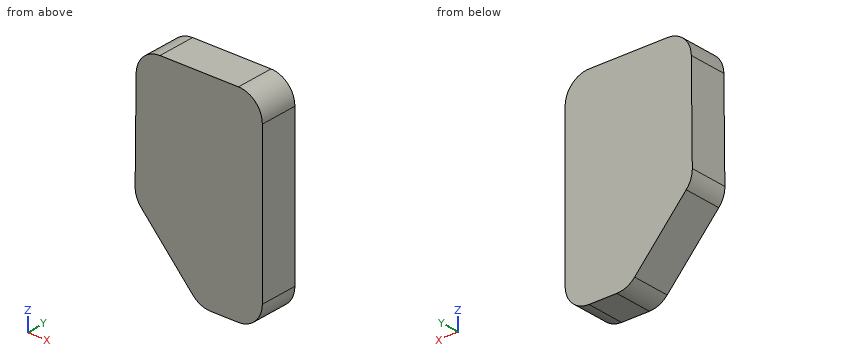
```python
from build123d import *

# Parameters (mm, degrees)
ESQUISSE1_W             = 80
ESQUISSE1_H             = 16
BOSS_EXTRU_1_DEPTH      = 85
ENL_V_MAT_EXTRU_1_DEPTH = 118.817655723
CONG_1_R                = 10
ENL_V_MAT_EXTRU_2_DEPTH = 118.817655723
CONG_2_R                = 10


with BuildPart() as part:
    # Esquisse1 → Boss.-Extru.1 (new body)
    with BuildSketch(Plane.XY):
        with Locations((40, 8)):
            Rectangle(ESQUISSE1_W, ESQUISSE1_H)
    extrude(amount=BOSS_EXTRU_1_DEPTH)

    # Esquisse4 → Enlèv. mat.-Extru.1 (cut, through all)
    with BuildSketch(Plane(origin=(0, 16, 0), x_dir=(1, 0, 0), z_dir=(0, 1, 0))):
        with BuildLine():
            Line((0, 0), (0, -60.067381304))
            Line((0, -60.067381304), (50.91884997, -3.321412558))
            ThreePointArc((50.91884997, -3.321412558), (54.286554034, -0.868026653), (58.361730446, 0))
            Line((58.361730446, 0), (0, 0))
        make_face()
    extrude(amount=-ENL_V_MAT_EXTRU_1_DEPTH, mode=Mode.SUBTRACT)

    # Congé1
    cong_1_edges = [part.edges().sort_by_distance(p)[0] for p in [
        (0, 8, 60.067381304),
    ]]
    fillet(cong_1_edges, radius=CONG_1_R)

    # Esquisse5 → Enlèv. mat.-Extru.2 (cut, through all)
    with BuildSketch(Plane(origin=(0, 0, 0), x_dir=(-1, 0, 0), z_dir=(0, -1, 0))):
        Polygon((-27.29979965, -85), (-26.737984747, -30.269519654), (25.961948545, -37.418966658), (23.023106213, -85), align=None)
    extrude(amount=-ENL_V_MAT_EXTRU_2_DEPTH, mode=Mode.SUBTRACT)

    # Congé2
    cong_2_edges = [part.edges().sort_by_distance(p)[0] for p in [
        (80, 8, 85),
        (27.29979965, 8, 85),
        (26.737984747, 8, 30.269519654),
        (80, 8, 0),
    ]]
    fillet(cong_2_edges, radius=CONG_2_R)


solid = part.part
```
Design review of the part built by this model. Coordinates are the model's own, in mm. Round coordinates to 2 decimals unless told otherwise and drop trailing zeros. Write each loop counter-clockwise with the first axis right and the second up, starting at its lowest first coordinate (ties: lowest second). Pieces come first, ordered by that corner, then holes.
Item 1: For probe 1 along X at (y, z) = (2.5, 74.5); probe 2 along Z at (x, y) = (70.5, 5); probe 3 along Z at (x, y) = (35, 10.25), list the stretches that pass through material, from the lowest coordinate up.
Item 2: Clearance check with a flat-ended pin moving along its axis: pin 1 Ø6 at (y, z) = (2.5, 62) entering from -X. State where the tip first meets the part, or that it passes through.
Item 3: We need section A-A on y = 10.25. Write out the cut boundary in (x, z).
Item 4: We need section C-C on z = 24. Write out the cut boundary in (x, y).
Item 5: We need section B-B on x = 39.5. Write out the cut boundary in (y, z), and give its area (3 significant figures).
Returned:
1. probe 1: x = 27.19 to 80
1. probe 2: z = 0.01 to 84.99
1. probe 3: z = 21.06 to 84.76
2. pin 1: stops at x = 27.03
3. outline: (26.78, 34.16) arc R10 ccw to (29.33, 27.38) - (50.92, 3.32) arc R10 ccw to (58.36, 0) - (70, 0) arc R10 ccw to (80, 10) - (80, 75) arc R10 ccw to (70, 85) - (37.2, 85) arc R10 ccw to (27.2, 75.1) - close
4. outline: (32.36, 0) - (80, 0) - (80, 16) - (32.36, 16) - close
5. outline: (0, 16.05) - (16, 16.05) - (16, 85) - (0, 85) - close
5. area: 1,100 mm2
